Could you check a few things on this model? Use its own coordinates, in mm. Give positions to 0.01 mm unless a question says otherwise; leave off trailing zeros. Loops run counter-clockwise (first coordinate to the right, second up) from the corner with the lowest first, then second, coordinate; pieces in that order, holes last.
1. I need wall thicknesses on line 1 along Z through (x, y) = (-167.5, -0.8) (3 decimals); line 2 along X through (y, z) = (-0.3, 126.5) (3 decimals); line 3 along X through (y, z) = (-0.3, -121.5) (3 decimals). Which ranges of each line are inside material? Lowest first, please.
2. For P1, Ø0.8, axis at x = -18.5, y = -0.5, coming from the +Z side; P2, Ø0.5, axis at x = -60, y = -0.5, coming from the -Z side; P3, Ø0.5, axis at y = -0.5, z = -9.5, coming from the -X side, each with a flat end and sliding along its axis, tell me the tip position at first contact or that it passes through.
3. Imagine slicing it at D-D (y = -1.05). Count the separate pieces of the cut face and the enclosed holes in it, plus the area to 3 significant figures.
4. Imagine slicing it at B-B (z = -52.5). List the corners of the cut face in (x, y) for me, plus the area to 3 significant figures.
5. Imagine slicing it at C-C (x = 58.5). List the corners of the cut face in (y, z) for me.
6. Imagine slicing it at A-A (x = 0). List the corners of the cut face in (y, z) for me, plus the area to 3 significant figures.
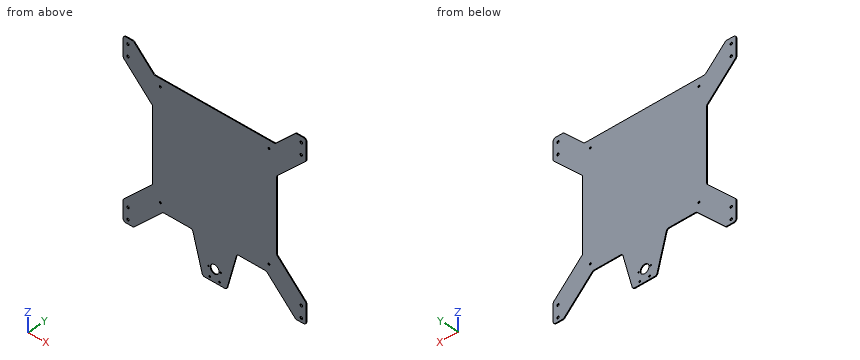
```python
from build123d import *

# Parameters (mm, degrees)
SKETCH1_W            = 350
SKETCH1_H            = 347
BASE_FLANGE1_DEPTH   = 1.51892
M3_CLEARANCE_HOLE1_D = 3.6
M4_CLEARANCE_HOLE1_D = 4.8
SKETCH13_R           = 8.5
SKETCH13_R_2         = 1.375
CUT_EXTRUDE1_DEPTH   = 1.51892
SKETCH41_W           = 347
SKETCH41_H           = 1.51892
BOSS_EXTRUDE4_DEPTH  = 1.905
SKETCH42_W           = 347
SKETCH42_H           = 1.51892
BOSS_EXTRUDE5_DEPTH  = 1.905
CUT_EXTRUDE2_DEPTH   = 1.51892
BOSS_EXTRUDE6_DEPTH  = 1.51892
CLEARANCE_HOLE2_D    = 3.4
FILLET2_R            = 5


# Sheet-metal steps are written as plain solids
with BuildPart() as part:
    # Sketch1 → Base-Flange1 (new body)
    with BuildSketch(Plane(origin=(0, 0, 0), x_dir=(1, 0, 0), z_dir=(0, 1, 0))):
        with Locations((0, 13.5)):
            Rectangle(SKETCH1_W, SKETCH1_H)
    extrude(amount=-BASE_FLANGE1_DEPTH)

    # M3 Clearance Hole1 (through all)
    with Locations(Plane(origin=(0, 0, 0), x_dir=(1, 0, 0), z_dir=(0, 1, 0))):
        with Locations((-105, 105), (105, 105), (105, -105), (-105, -105)):
            Hole(M3_CLEARANCE_HOLE1_D / 2)

    # M4 Clearance Hole1 (through all)
    with Locations(Plane(origin=(0, -1.51892, 0), x_dir=(-1, 0, 0), z_dir=(0, -1, 0))):
        with Locations((167.5, 146.5), (167.5, 169), (-167.5, 146.5), (-167.5, 169), (-167.5, -149), (-167.5, -126.5), (167.5, -149), (167.5, -126.5)):
            Hole(M4_CLEARANCE_HOLE1_D / 2)

    # Sketch13 → Cut-Extrude1 (cut)
    with BuildSketch(Plane(origin=(0, 0, 0), x_dir=(1, 0, 0), z_dir=(0, 1, 0))):
        with Locations(Location((0, 170, 0), (0, 0, 270))):
            Circle(SKETCH13_R)
        with Locations(Location((-11.825, 170, 0), (0, 0, 270))):
            Circle(SKETCH13_R_2)
        with Locations(Location((11.825, 170, 0), (0, 0, 270))):
            Circle(SKETCH13_R_2)
    extrude(amount=-CUT_EXTRUDE1_DEPTH, mode=Mode.SUBTRACT)

    # Sketch41 → Boss-Extrude4 (add)
    with BuildSketch(Plane(origin=(175, 0, 0), x_dir=(0, 0, -1), z_dir=(1, 0, 0))):
        with Locations((13.5, -0.75946)):
            Rectangle(SKETCH41_W, SKETCH41_H)
    extrude(amount=BOSS_EXTRUDE4_DEPTH)

    # Sketch42 → Boss-Extrude5 (add)
    with BuildSketch(Plane.ZY.offset(175)):
        with Locations((-13.5, -0.75946)):
            Rectangle(SKETCH42_W, SKETCH42_H)
    extrude(amount=BOSS_EXTRUDE5_DEPTH)

    # Sketch43 → Cut-Extrude2 (cut)
    with BuildSketch(Plane(origin=(0, 0, 0), x_dir=(1, 0, 0), z_dir=(0, 1, 0))):
        Polygon((-176.905, -120), (-120, -63.095), (-120, 80.095), (-176.905, 137), align=None)
        Polygon((-156.905, 177), (-99.905, 120), (-42.952595893, 120), (-25, 187), (-176.905, 187), (-176.905, 177), align=None)
        Polygon((25, 187), (42.952595893, 120), (99.905, 120), (156.905, 177), (176.905, 177), (176.905, 187), align=None)
        Polygon((120, 80.095), (120, -63.095), (176.905, -120), (176.905, 137), align=None)
        Polygon((116.905, -120), (-116.905, -120), (-156.905, -160), (156.905, -160), align=None)
    extrude(amount=-CUT_EXTRUDE2_DEPTH, mode=Mode.SUBTRACT)

    # Sketch45 → Boss-Extrude6 (add)
    with BuildSketch(Plane(origin=(0, 0, 0), x_dir=(1, 0, 0), z_dir=(0, 1, 0))):
        Polygon((-25, 187), (-23.124355653, 194), (23.124355653, 194), (25, 187), align=None)
    extrude(amount=-BOSS_EXTRUDE6_DEPTH)

    # Clearance Hole2 (through all)
    with Locations(Plane(origin=(0, 0, 0), x_dir=(1, 0, 0), z_dir=(0, 1, 0))):
        with Locations((-9.525, 188), (9.525, 188)):
            Hole(CLEARANCE_HOLE2_D / 2)

    # Fillet2
    fillet2_edges = [part.edges().sort_by_distance(p)[0] for p in [
        (176.905, -0.75946, 160),
        (-176.905, -0.75946, 160),
        (176.905, -0.75946, -177),
        (42.952595893, -0.75946, -120),
        (99.905, -0.75946, -120),
        (156.905, -0.75946, -177),
        (176.905, -0.75946, 120),
        (176.905, -0.75946, -137),
        (120, -0.75946, -80.095),
        (120, -0.75946, 63.095),
        (-176.905, -0.75946, -137),
        (-176.905, -0.75946, 120),
        (-120, -0.75946, 63.095),
        (-120, -0.75946, -80.095),
        (-176.905, -0.75946, -177),
        (-156.905, -0.75946, -177),
        (-99.905, -0.75946, -120),
        (-42.952595893, -0.75946, -120),
        (-156.905, -0.75946, 160),
        (156.905, -0.75946, 160),
        (116.905, -0.75946, 120),
        (-116.905, -0.75946, 120),
        (-23.124355653, -0.75946, -194),
        (23.124355653, -0.75946, -194),
    ]]
    fillet(fillet2_edges, radius=FILLET2_R)


solid = part.part
```
Derived:
1. line 1: z = -177 to -171.4, -166.6 to -148.9, -144.1 to -127.595, 110.595 to 124.1, 128.9 to 146.6, 151.4 to 160
1. line 2: x = -176.905 to -169.9, -165.1 to -123.405, 123.405 to 165.1, 169.9 to 176.905
1. line 3: x = -161.405 to -101.405, -43.219 to 43.219, 101.405 to 161.405
2. P1: stops at z = 120
2. P2: stops at z = -120
2. P3: stops at x = -120
3. separate pieces: 1
3. enclosed holes: 17
3. area: 75,300 mm2
4. outline: (-120, -1.52) - (120, -1.52) - (120, 0) - (-120, 0) - close
4. area: 365 mm2
5. outline: (-1.52, -120) - (0, -120) - (0, 120) - (-1.52, 120) - close
6. outline: (-1.52, -194) - (0, -194) - (0, -178.5) - (-1.52, -178.5) - close; (-1.52, -161.5) - (0, -161.5) - (0, 120) - (-1.52, 120) - close
6. area: 451 mm2
